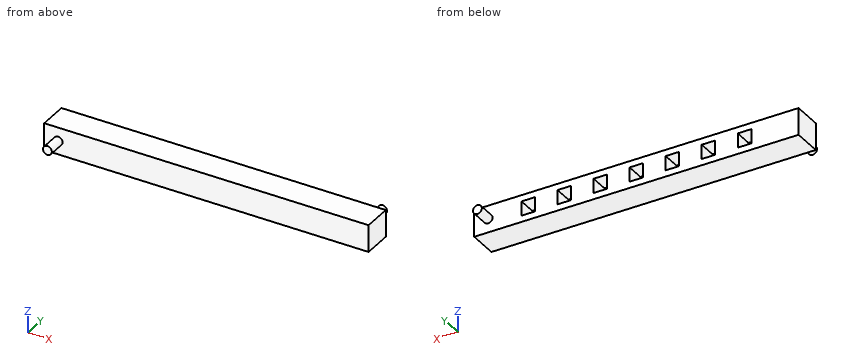
```python
from build123d import *

# Parameters (mm, degrees)
F0_W     = 228.6
F0_H     = 19.05
F1_DEPTH = 20.32
F3_W     = 9.525
F3_H     = 10.16
F4_DEPTH = 12.7
F2_R     = 3.1115
F5_DEPTH = 12.7
F6_R     = 3.1115
F7_DEPTH = 12.7


with BuildPart() as f1:
    # F0 (on Front) → F1 (new body)
    with BuildSketch(Plane.XZ):
        Rectangle(F0_W, F0_H)
    extrude(amount=F1_DEPTH)

    # F3 (on face) → F4 (cut)
    with BuildSketch(Plane(origin=(0, 0, 0), x_dir=(-1, 0, 0), z_dir=(0, 1, 0))):
        Rectangle(F3_W, F3_H)
        with Locations((25.4, 0)):
            Rectangle(F3_W, F3_H)
        with Locations((50.8, 0)):
            Rectangle(F3_W, F3_H)
        with Locations((-25.4, 0)):
            Rectangle(F3_W, F3_H)
        with Locations((-50.8, 0)):
            Rectangle(F3_W, F3_H)
        with Locations((-76.2, 0)):
            Rectangle(F3_W, F3_H)
        with Locations((76.2, 0)):
            Rectangle(F3_W, F3_H)
    extrude(amount=-F4_DEPTH, mode=Mode.SUBTRACT)

    # F2 (on face) → F5 (join)
    with BuildSketch(Plane.XZ.offset(20.32)):
        with Locations((-104.4829, 0)):
            Circle(F2_R)
    extrude(amount=F5_DEPTH)

    # F6 (on face) → F7 (join)
    with BuildSketch(Plane(origin=(0, 0, 0), x_dir=(-1, 0, 0), z_dir=(0, 1, 0))):
        with Locations((-104.4829, 0)):
            Circle(F6_R)
    extrude(amount=F7_DEPTH)


solid = f1.part
```
Verification items for the finished model (mm, model axes). Round coordinates to 2 decimals unless told otherwise and drop trailing zeros. Write each loop counter-clockwise with the first axis right and the second up, starting at its lowest first coordinate (ties: lowest second). Pieces come first, ordered by that corner, then holes.
1. Section check B-B on x = 74. Enter the section's corners in (y, z) (3 decimals), plus the area to 3 significant figures.
2. Gauge pin test, flat end, axial feed: P1, Ø10.5, axis at x = -49.5, z = 1, coming from the +Y side. Record the tip position at first contact, or that the pin passes through.
3. Scan lines: L1, parallel to Y at x = 29, z = 5.5; L2, parallel to Y at x = -28.5, z = 2.75; L3, parallel to X at y = -26, z = -1.25. Record each from-to range of solid material in increasing order.
4. Section check D-D on x = -38. Enter the section's corners in (y, z) (3 decimals).
5. Section check A-A on y = -4.5. State how many separate pieces and enclosed holes the cut face has, plus the area to 3 significant figures.
6. Section check C-C on z = 7.25. Enter the section's corners in (x, y).
Answer:
1. outline: (-20.32, -9.525) - (0, -9.525) - (0, -5.08) - (-12.7, -5.08) - (-12.7, 5.08) - (0, 5.08) - (0, 9.525) - (-20.32, 9.525) - close
1. area: 258 mm2
2. P1: stops at y = 0
3. L1: y = -20.32 to 0
3. L2: y = -20.32 to -12.7
3. L3: x = -107.33 to -101.63
4. outline: (-20.32, -9.525) - (0, -9.525) - (0, 9.525) - (-20.32, 9.525) - close
5. separate pieces: 1
5. enclosed holes: 7
5. area: 3,680 mm2
6. outline: (-114.3, -20.32) - (114.3, -20.32) - (114.3, 0) - (-114.3, 0) - close
